Read the model definition and answer for the solid it produces. Units are mm, in the model's axes. Face numbers are marked on the shaded views. A direction names the side the tool comes from. Coordinates: 2 decimals unless noted, no trailing zeros. Write each loop counter-clockwise with the first axis right and the second up, starting at its lowest first coordinate (ties: lowest second). Pieces come first, ordered by that corner, then holes. Notation, with made-up numbers: (2, 32.25) - (38, 32.25) arc R21 ccw to (38, 68.25) - close; hole circle Ø11 at (49.25, 37.5). An arc over 180 degrees is marked (long way). Use a Markdown table: item, result.
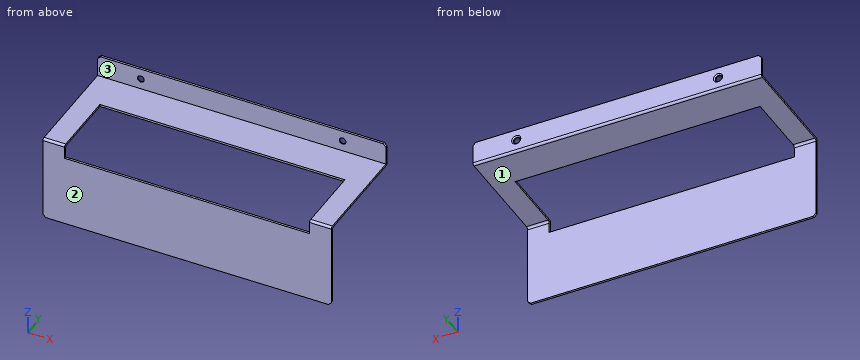
from build123d import *

# Parameters (mm, degrees)
F1_DEPTH       = 200
F2_SIZE        = 2
F4_D           = 4.7
F4_CSINK_D     = 6.3
F4_CSINK_ANGLE = 90
F6_DEPTH       = 10
F7_R           = 1.5


with BuildPart() as f1:
    # F0 (on Right) → F1 (new body)
    with BuildSketch(Plane.YZ):
        Polygon((25.307591, 44.168082), (-48.192409, 44.168082), (-48.192409, -15.831918), (-46.692409, -15.831918), (-46.692409, 42.668082), (26.807591, 42.668082), (26.807591, 44.168082), (26.807591, 59.168082), (25.307591, 59.168082), align=None)
    extrude(amount=F1_DEPTH)

    # F2
    f2_edges = [f1.edges().sort_by_distance(p)[0] for p in [
        (200, 26.057591, 59.168082),
        (0, 26.057591, 59.168082),
        (0, -47.442409, -15.831918),
        (200, -47.442409, -15.831918),
    ]]
    chamfer(f2_edges, length=F2_SIZE)

    # F4 (through all)
    with Locations(Plane(origin=(0, 26.807591, 0), x_dir=(-1, 0, 0), z_dir=(0, 1, 0))):
        with Locations((-170, 51.668082), (-30, 51.668082)):
            CounterSinkHole(F4_D / 2, F4_CSINK_D / 2, counter_sink_angle=F4_CSINK_ANGLE)

    # F5 (on face) → F6 (cut)
    with BuildSketch(Plane.XY.offset(44.168082)):
        Polygon((185, -53.390387), (185, -0.692409), (15, -0.692409), (15, -52.513979), align=None)
    extrude(amount=-F6_DEPTH, mode=Mode.SUBTRACT)

    # F7
    f7_edges = [f1.edges().sort_by_distance(p)[0] for p in [
        (7.5, -48.192409, 44.168082),
        (192.5, -48.192409, 44.168082),
        (100, 26.807591, 42.668082),
        (192.5, -46.692409, 42.668082),
        (7.5, -46.692409, 42.668082),
    ]]
    fillet(f7_edges, radius=F7_R)


solid = f1.part
(1) A cutting plane is placed at C-C, the plane x = 30. Write down the section's boundary in (y, z), and give its area (3 significant figures).
Report:
| item | result |
|---|---|
| outline | (-48.19, -15.83) - (-46.69, -15.83) - (-46.69, 34.17) - (-48.19, 34.17) - close; (-0.69, 42.67) - (25.31, 42.67) arc R1.5 ccw to (26.81, 44.17) - (26.81, 48.52) - (26.01, 49.32) - (25.31, 49.32) - (25.31, 44.17) - (-0.69, 44.17) - close; (25.31, 54.02) - (26.01, 54.02) - (26.81, 54.82) - (26.81, 59.17) - (25.31, 59.17) - close |
| area | 131 mm² |
(2) A cutting plane is placed at D-D, the plane z = 31. Write down the section's boundary in (x, y), and give its area (3 significant figures).
Report:
| item | result |
|---|---|
| outline | (0, -48.19) - (200, -48.19) - (200, -46.69) - (0, -46.69) - close |
| area | 300 mm² |
(3) Each of these flat-tipped pins is pushed along its axis until it touches: P1, Ø12, axis at x = 133.5, z = 54, coming from the -Y side; P2, Ø12, axis at x = 136.5, z = 47, coming from the -Y side. Where does it stop, or does it pass through?
Report:
| item | result |
|---|---|
| P1 | stops at y = 25.31 |
| P2 | stops at y = -0.69 |
(4) A cutting plane is placed at A-A, the plane x = 100. Write down the section's boundary in (y, z), and give its area (3 significant figures).
Report:
| item | result |
|---|---|
| outline | (-48.19, -15.83) - (-46.69, -15.83) - (-46.69, 34.17) - (-48.19, 34.17) - close; (-0.69, 42.67) - (25.31, 42.67) arc R1.5 ccw to (26.81, 44.17) - (26.81, 59.17) - (25.31, 59.17) - (25.31, 44.17) - (-0.69, 44.17) - close |
| area | 138 mm² |
(5) For the marked faces 1, 2 and 3, determine the directions among +Z, -Z, +X, -X, +Y, -Y from which every point of the face is accessible in a straight line to the end or side of a thin tool.
Report:
| item | result |
|---|---|
| face 1 | -Z, +X, -X, +Y |
| face 2 | +Z, -Z, +X, -X, -Y |
| face 3 | +Z, +X, -X, -Y |
(6) A cutting plane is placed at B-B, the plane y = -31. Write down the section's boundary in (x, z), and give its area (3 significant figures).
Report:
| item | result |
|---|---|
| outline | (0, 42.67) - (15, 42.67) - (15, 44.17) - (0, 44.17) - close; (185, 42.67) - (200, 42.67) - (200, 44.17) - (185, 44.17) - close |
| area | 45.0 mm² |
(7) Straight lines are drawn through the part: L1, parallel to Y at x = 101, z = -8; L2, parallel to Z at x = 170, y = 25; L3, parallel to Z at x = 170, y = 25.7. For each, find the intervals that lie inside material, in ascending order.
Report:
| item | result |
|---|---|
| L1 | y = -48.19 to -46.69 |
| L2 | z = 42.67 to 44.17 |
| L3 | z = 42.72 to 49.32, 54.02 to 59.17 |
